The model under review builds one solid part; all positions refer to its coordinate system, in mm. Give positions to 0.01 mm unless a question says otherwise; leave off trailing zeros. Order: outer loops, then holes, each group sorted by start corner. A loop starts at its lowest first (then second) coordinate and runs counter-clockwise, first axis right, second up.
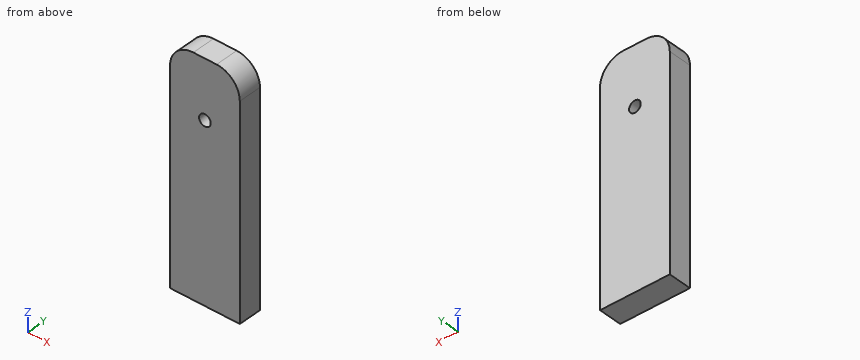
```python
from build123d import *

# Parameters (mm, degrees)
F0_W     = 76.2
F0_H     = 25.4
F1_DEPTH = 254
F2_R     = 25.4
F4_D     = 12.7


with BuildPart() as f1:
    # F0 (on Top) → F1 (new body)
    with BuildSketch(Plane.XY):
        with Locations((38.1, 41.066651)):
            Rectangle(F0_W, F0_H)
    extrude(amount=F1_DEPTH)

    # F2
    f2_edges = [f1.edges().sort_by_distance(p)[0] for p in [
        (0, 41.066651, 254),
        (76.2, 41.066651, 254),
    ]]
    fillet(f2_edges, radius=F2_R)

    # F4 (through all)
    with Locations(Plane(origin=(0, 53.766651, 0), x_dir=(-1, 0, 0), z_dir=(0, 1, 0))):
        with Locations((-38.1, 190.5)):
            Hole(F4_D / 2)


solid = f1.part
```
Item 1: Take a section at D-D (x = 11.5). Give the boundary of the cut face in (y, z), and give its area (3 significant figures).
Values found:
outline: (28.37, 0) - (53.77, 0) - (53.77, 249.86) - (28.37, 249.86) - close
area: 6,350 mm2
Item 2: Take a section at A-A (x = 38.1). Give the boundary of the cut face in (y, z).
Values found:
outline: (28.37, 0) - (53.77, 0) - (53.77, 184.15) - (28.37, 184.15) - close; (28.37, 196.85) - (53.77, 196.85) - (53.77, 254) - (28.37, 254) - close
Item 3: Clearance check with a flat-ended pin moving along its axis: pin 1 Ø1 at (x, y) = (20.5, 37.5) entering from +Z. State where the tip first meets the part, or that it passes through.
Values found:
pin 1: stops at z = 253.62
Item 4: Take a section at B-B (z = 190.5). Give the boundary of the cut face in (x, y), and give its area (3 significant figures).
Values found:
outline: (0, 28.37) - (31.75, 28.37) - (31.75, 53.77) - (0, 53.77) - close; (44.45, 28.37) - (76.2, 28.37) - (76.2, 53.77) - (44.45, 53.77) - close
area: 1,610 mm2
Item 5: For line 1 (Z direction, x = 38.1, y = 45.5); line 2 (Z direction, x = 35, y = 48.5); line 3 (X direction, y = 48.25, z = 234.5), list the stretches that pass through material, from the lowest coordinate up.
Values found:
line 1: z = 0 to 184.15, 196.85 to 254
line 2: z = 0 to 184.96, 196.04 to 254
line 3: x = 0.69 to 75.51
Item 6: Take a section at C-C (y = 49). Give the boundary of the cut face in (x, z).
Values found:
outline: (0, 0) - (76.2, 0) - (76.2, 228.6) arc R25.4 ccw to (50.8, 254) - (25.4, 254) arc R25.4 ccw to (0, 228.6) - close; hole circle Ø12.7 at (38.1, 190.5)
